Drawing for the job (mm, zero at the part's lowest x, y, z). Coordinates: 2 decimals unless noted, no trailing zeros. Loops run counter-clockwise (first coordinate to the right, second up) from the corner with the lowest first, then second, coordinate; pieces in that order, holes last.
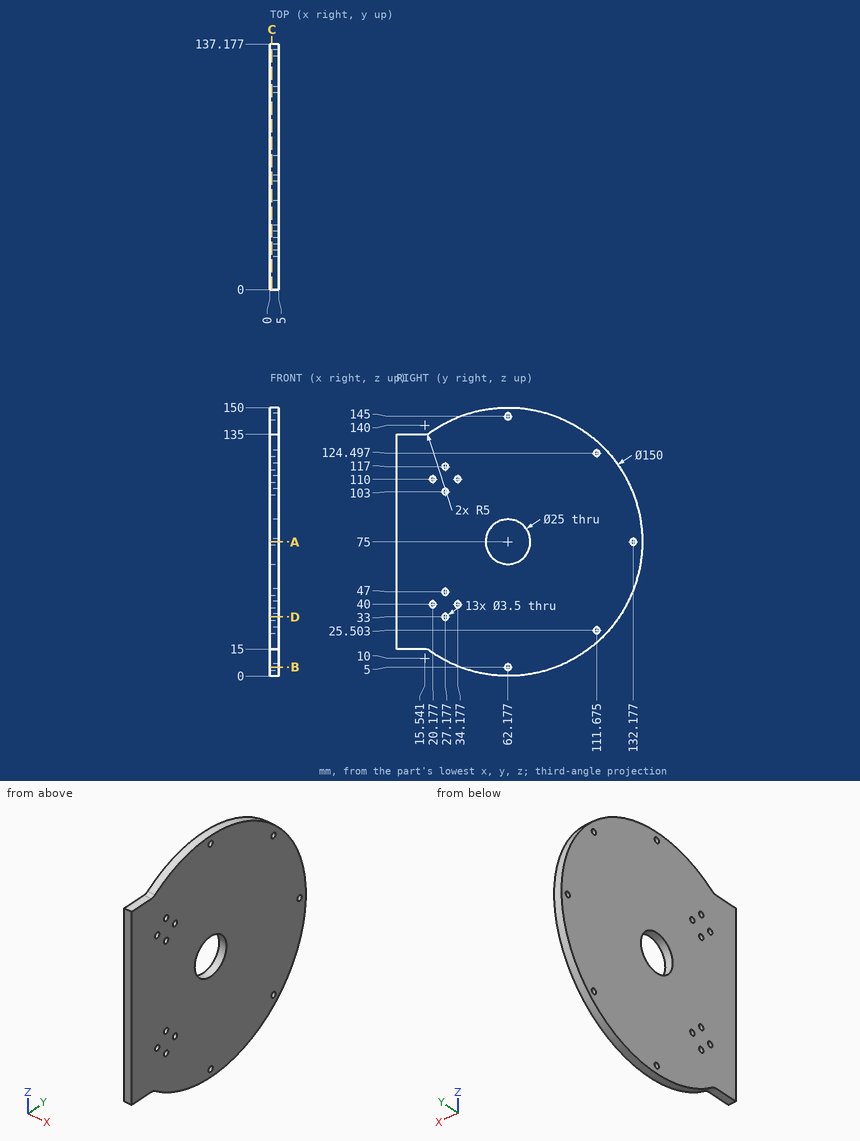
Q1. Drop flat-ended pins along their axis: P1, Ø3, axis at y = 27.18, z = 33, coming from the +X side; P2, Ø2.5, axis at x = 2.5, y = 8, coming from the -Z side; P3, Ø1.5, axis at x = 1.5, y = 115, coming from the +Z side (1 decimal); P4, Ø2, axis at x = 1.5, y = 46, coming from the +Z side. Give the stop position or say it passes through.
Q2. Saw through at A-A (z = 75). List the corners of the cut face in (x, y).
Q3. Saw through at D-D (z = 33). List the corners of the cut face in (x, y) (1 decimal), plus the area to 3 significant figures.
Q4. Probe line 1 (Z direction, x = 3.4, y = 63) (1 decimal); line 2 (Z direction, x = 1.4, y = 113) (1 decimal); line 3 (Y direction, x = 1.7, z = 40). List the from-to ranges inside material, lowest first.
Q5. Saw through at C-C (x = 1.2). Count the separate pieces of the cut face and the enclosed holes in it, plus the area to 3 significant figures.
Q6. Saw through at B-B (z = 5). List the corners of the cut face in (x, y).
Checked values:
1. P1: passes through
1. P2: stops at z = 15
1. P3: stops at z = 129
1. P4: stops at z = 148.45
2. outline: (0, 0) - (5, 0) - (5, 49.68) - (0, 49.68) - close; (0, 74.68) - (5, 74.68) - (5, 130.43) - (0, 130.43) - close; (0, 133.93) - (5, 133.93) - (5, 137.18) - (0, 137.18) - close
3. outline: (0, 0) - (5, 0) - (5, 25.4) - (0, 25.4) - close; (0, 28.9) - (5, 28.9) - (5, 124.3) - (0, 124.3) - close
3. area: 604 mm2
4. line 1: z = 0 to 3.5, 6.5 to 62.5, 87.5 to 143.5, 146.5 to 150
4. line 2: z = 19.8 to 24.4, 26.6 to 123.4, 125.6 to 130.2
4. line 3: y = 0 to 18.43, 21.93 to 32.43, 35.93 to 128.51
5. separate pieces: 1
5. enclosed holes: 14
5. area: 16,600 mm2
6. outline: (0, 35.25) - (5, 35.25) - (5, 60.43) - (0, 60.43) - close; (0, 63.93) - (5, 63.93) - (5, 89.1) - (0, 89.1) - close
